Here's how the part is built. I have some questions about the finished solid (model axes, mm). A direction names the side the tool comes from. Coordinates: 2 decimals unless noted, no trailing zeros. Order: outer loops, then holes, each group sorted by start corner. A loop starts at its lowest first (then second) coordinate and runs counter-clockwise, first axis right, second up. Notation, with made-up numbers: (30, 35.5) - (71, 35.5) arc R24 cw to (71, 63.5) - close; hole circle Ø2 at (62.5, -1). An arc over 180 degrees is marked (long way). Answer in a Markdown table with one row per item. Add a question column.
Item 1: Thinking about a two-plate mould opening in Y: for faces 1 (the flat face through (6, 5.766, 3)), 2 (the flat face through (0.635, 3, 4)), 3 (the flat face through (0.9, 5.4, 6.985)), which applies, +Y half, -Y half, draft (parallel to the pull), parting line (faces both ways), or undercut?
Item 2: Will these pins go through, and if not, where does the flat tip stop? pin 1 Ø1.5 at (x, y) = (2.5, 1) entering from +Z (3 decimals); pin 2 Ø0.5 at (x, y) = (7.5, 3.5) entering from +Z; pin 3 Ø0.7 at (x, z) = (10, -1.5) entering from -Y; pin 4 Ø0.5 at (y, z) = (3.5, -2.5) entering from -X.
Item 3: If I drill on line 1 along X through (y, z) = (3.3, 4) (1 decimal); line 2 along Y through (x, z) = (5, 1.5) (3 decimals); line 3 along X through (y, z) = (3.7, -0.25), over which ranges is the centre line in solid material (lowest first)? Write a range as from..to.
Item 4: I want a section at A-A (z = 2). Please give me the cut outline in (x, y) (1 decimal).
Item 5: I want a section at C-C (y = 5.3). Please give me the cut outline in (x, z) (3 decimals), plus the area to 3 significant figures.
Item 6: I want a section at B-B (z = -2). Please give me the cut outline in (x, y), plus the area to 3 significant figures.
Item 7: I want a section at D-D (x = 1.5). Please give me the cut outline in (y, z) (3 decimals), plus the area to 3 significant figures.
Item 8: On a 3-axis mill with a long thin cutter (end or side, diameter ignored), from which of +Z, -Z, +X, -X, +Y, -Y can I reach the whole of each face in a straight line? I mean faces 4 (the flat face through (11.786, 3, 4)), 5 (the flat face through (0, 3, 3)). Say none if no direction works.
```python
from build123d import *

# Parameters (mm, degrees)
SKETCH1_W           = 12.4206
SKETCH1_H           = 5.7658
BOSS_EXTRUDE1_DEPTH = 6.985
SKETCH2_W           = 0.6604
SKETCH2_H           = 0.6604
BOSS_EXTRUDE2_DEPTH = 3.175
SKETCH4_W           = 11.1506
SKETCH4_H           = 4.4958
CUT_EXTRUDE1_DEPTH  = 6.35
SKETCH2_2_W         = 0.6604
SKETCH2_2_H         = 0.6604
BOSS_EXTRUDE3_DEPTH = 6.35
SKETCH5_W           = 0.635
SKETCH5_H           = 1.016
SKETCH5_W_2         = 1.524
SKETCH5_H_2         = 0.635
CUT_EXTRUDE2_DEPTH  = 3.556


with BuildPart() as part:
    # Sketch1 → Boss-Extrude1 (new body)
    with BuildSketch(Plane.XY):
        with Locations((6.2103, 2.8829)):
            Rectangle(SKETCH1_W, SKETCH1_H)
    extrude(amount=BOSS_EXTRUDE1_DEPTH)

    # Sketch2 → Boss-Extrude2 (add)
    with BuildSketch(Plane(origin=(0, 0, 0), x_dir=(-1, 0, 0), z_dir=(0, 0, -1))):
        with Locations((-9.9603, 3.4036)):
            Rectangle(SKETCH2_W, SKETCH2_H)
        with Locations((-7.4603, 3.4036)):
            Rectangle(SKETCH2_W, SKETCH2_H)
        with Locations((-4.9603, 3.4036)):
            Rectangle(SKETCH2_W, SKETCH2_H)
        with Locations((-2.4603, 3.4036)):
            Rectangle(SKETCH2_W, SKETCH2_H)
    extrude(amount=BOSS_EXTRUDE2_DEPTH)

    # Sketch4 → Cut-Extrude1 (cut)
    with BuildSketch(Plane.XY.offset(6.985)):
        with Locations((6.2103, 2.8829)):
            Rectangle(SKETCH4_W, SKETCH4_H)
    extrude(amount=-CUT_EXTRUDE1_DEPTH, mode=Mode.SUBTRACT)

    # Sketch2<2> → Boss-Extrude3 (add)
    with BuildSketch(Plane(origin=(0, 0, 0), x_dir=(-1, 0, 0), z_dir=(0, 0, -1))):
        with Locations((-9.9603, 3.4036)):
            Rectangle(SKETCH2_2_W, SKETCH2_2_H)
        with Locations((-7.4603, 3.4036)):
            Rectangle(SKETCH2_2_W, SKETCH2_2_H)
        with Locations((-4.9603, 3.4036)):
            Rectangle(SKETCH2_2_W, SKETCH2_2_H)
        with Locations((-2.4603, 3.4036)):
            Rectangle(SKETCH2_2_W, SKETCH2_2_H)
    extrude(amount=-BOSS_EXTRUDE3_DEPTH)

    # Sketch5 → Cut-Extrude2 (cut)
    with BuildSketch(Plane.XY.offset(6.985)):
        with Locations((0.3175, 4.3688)):
            Rectangle(SKETCH5_W, SKETCH5_H)
        with Locations((12.1031, 4.3688)):
            Rectangle(SKETCH5_W, SKETCH5_H)
        with Locations((9.7663, 5.4483)):
            Rectangle(SKETCH5_W_2, SKETCH5_H_2)
        with Locations((2.6543, 5.4483)):
            Rectangle(SKETCH5_W_2, SKETCH5_H_2)
    extrude(amount=-CUT_EXTRUDE2_DEPTH, mode=Mode.SUBTRACT)


solid = part.part
```
Values follow:
| question | item | result |
|---|---|---|
| 1 | face 1 | +Y half |
| 1 | face 2 | undercut |
| 1 | face 3 | draft |
| 2 | pin 1 | stops at z = 6.985 |
| 2 | pin 2 | stops at z = 6.35 |
| 2 | pin 3 | stops at y = 3.07 |
| 2 | pin 4 | stops at x = 2.13 |
| 3 | line 1 | x = 0..0.6, 2.1..2.8, 4.6..5.3, 7.1..7.8, 9.6..10.3, 11.8..12.4 |
| 3 | line 2 | y = 0..0.635, 3.073..3.734, 5.131..5.766 |
| 3 | line 3 | x = 2.13..2.79, 4.63..5.29, 7.13..7.79, 9.63..10.29 |
| 4 | outline | (0, 0) - (12.4, 0) - (12.4, 5.8) - (0, 5.8) - close; (2.1, 3.1) - (2.8, 3.1) - (2.8, 3.7) - (2.1, 3.7) - close; (4.6, 3.1) - (5.3, 3.1) - (5.3, 3.7) - (4.6, 3.7) - close; (7.1, 3.1) - (7.8, 3.1) - (7.8, 3.7) - (7.1, 3.7) - close; (9.6, 3.1) - (10.3, 3.1) - (10.3, 3.7) - (9.6, 3.7) - close; hole (0.6, 0.6) - (11.8, 0.6) - (11.8, 5.1) - (0.6, 5.1) - close |
| 5 | outline | (0, 0) - (12.421, 0) - (12.421, 6.985) - (10.528, 6.985) - (10.528, 3.429) - (9.004, 3.429) - (9.004, 6.985) - (3.416, 6.985) - (3.416, 3.429) - (1.892, 3.429) - (1.892, 6.985) - (0, 6.985) - close |
| 5 | area | 75.9 mm^2 |
| 6 | outline | (2.13, 3.07) - (2.79, 3.07) - (2.79, 3.73) - (2.13, 3.73) - close; (4.63, 3.07) - (5.29, 3.07) - (5.29, 3.73) - (4.63, 3.73) - close; (7.13, 3.07) - (7.79, 3.07) - (7.79, 3.73) - (7.13, 3.73) - close; (9.63, 3.07) - (10.29, 3.07) - (10.29, 3.73) - (9.63, 3.73) - close |
| 6 | area | 1.74 mm^2 |
| 7 | outline | (0, 0) - (5.766, 0) - (5.766, 6.985) - (5.131, 6.985) - (5.131, 0.635) - (0.635, 0.635) - (0.635, 6.985) - (0, 6.985) - close |
| 7 | area | 11.7 mm^2 |
| 8 | face 4 | +Z |
| 8 | face 5 | +Z, -Z, -X, +Y, -Y |
